Design review of the part shown in the three views and the two pictorial views. Dimensions are in mm from the part's minimum x, y and z. A direction names the side the tool comes from. Coordinates: 2 decimals unless noted, no trailing zeros. Loops run counter-clockwise (first coordinate to the right, second up) from the corner with the lowest first, then second, coordinate; pieces in that order, holes last. Notation, with made-up numbers: (84.25, 19.25) -> (96.25, 19.25) arc R4 ccw to (96.25, 25.25) -> close; hole circle Ø4 at (88.25, -25.75). An arc over 180 degrees is marked (long way). Answer in a Markdown table with one row per item.
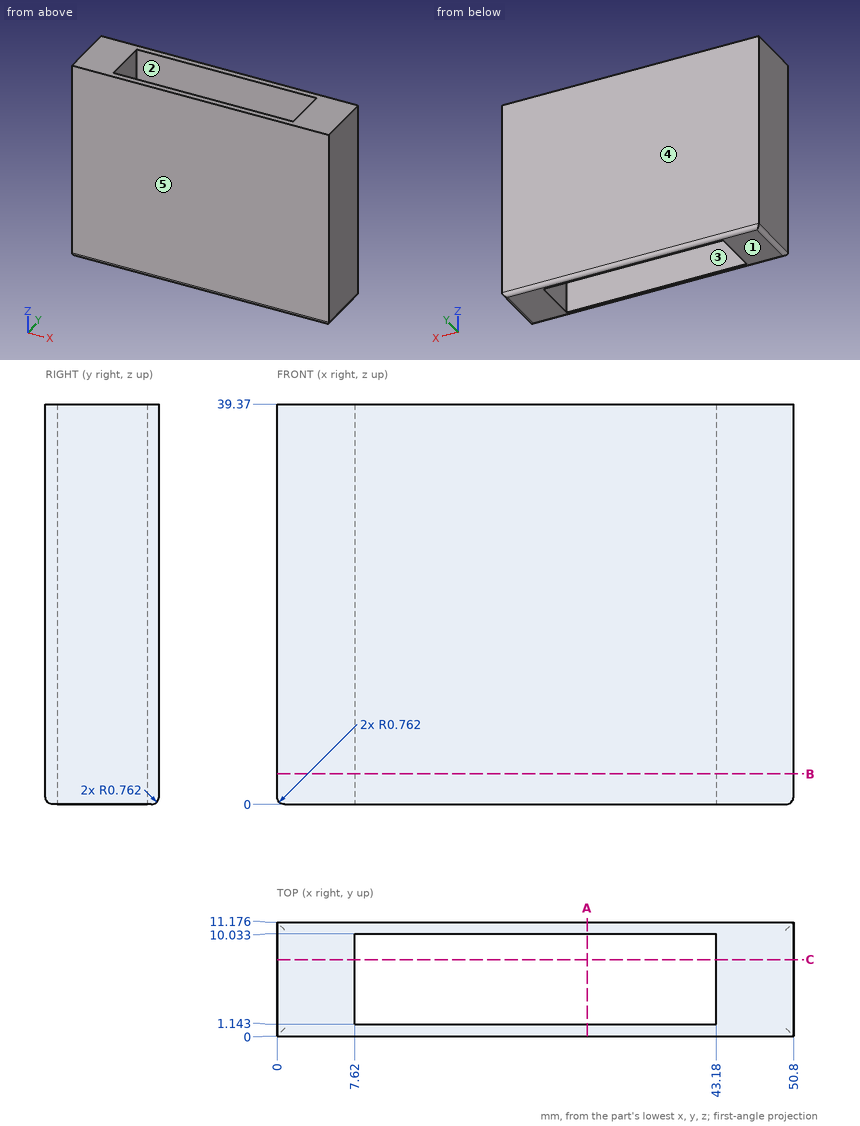
(1) Take a section at B-B on z = 3. Give the boundary of the cut face in (x, y), and give its area (3 significant figures).
Evaluation:
| item | result |
|---|---|
| outline | (0, 0) -> (50.8, 0) -> (50.8, 11.18) -> (0, 11.18) -> close; hole (7.62, 1.14) -> (43.18, 1.14) -> (43.18, 10.03) -> (7.62, 10.03) -> close |
| area | 252 mm² |
(2) Draft analysis for pull direction Y (two halves, no side actions). For the marked faces 3, 4 and 5, state which applies: pulls with the +Y half, pulls with the -Y half, needs draft (parallel to the pull), parting line crosses it, or undercut.
Evaluation:
| item | result |
|---|---|
| face 3 | undercut |
| face 4 | pulls with the +Y half |
| face 5 | pulls with the -Y half |
(3) To check wall thickness, follow probe 1 along X at (y, z) = (5.25, 26); probe 2 along Y at (x, z) = (18.5, 32.5); probe 3 along Z at (x, y) = (28.5, 10.75). State the ranges of each line that lie inside material, in increasing order.
Evaluation:
| item | result |
|---|---|
| probe 1 | x = 0 to 7.62, 43.18 to 50.8 |
| probe 2 | y = 0 to 1.14, 10.03 to 11.18 |
| probe 3 | z = 0.08 to 39.37 |
(4) Take a section at C-C on y = 7.5. Give the boundary of the cut face in (x, z), and give its area (3 significant figures).
Evaluation:
| item | result |
|---|---|
| outline | (0, 0.76) arc R0.76 ccw to (0.76, 0) -> (7.62, 0) -> (7.62, 39.37) -> (0, 39.37) -> close; (43.18, 0) -> (50.04, 0) arc R0.76 ccw to (50.8, 0.76) -> (50.8, 39.37) -> (43.18, 39.37) -> close |
| area | 600 mm² |
(5) Tool access review of the marked faces 1 and 2: name each direction out of +Z, -Z, +X, -X, +Y, -Y from which nothing blocks a thin tool from reaching the whole face with its end or side.
Evaluation:
| item | result |
|---|---|
| face 1 | -Z, +X, -X, +Y, -Y |
| face 2 | +Z, -Z |
(6) Take a section at A-A on x = 30.5. Give the boundary of the cut face in (y, z), and give its area (3 significant figures).
Evaluation:
| item | result |
|---|---|
| outline | (0, 0.76) arc R0.76 ccw to (0.76, 0) -> (1.14, 0) -> (1.14, 39.37) -> (0, 39.37) -> close; (10.03, 0) -> (10.41, 0) arc R0.76 ccw to (11.18, 0.76) -> (11.18, 39.37) -> (10.03, 39.37) -> close |
| area | 89.8 mm² |
